Geometry: final body of the model. Coordinates: model frame, mm. Face numbers are marked on the shaded views. A direction names the side the tool comes from. Round coordinates to 2 decimals unless told otherwise and drop trailing zeros. Write each loop counter-clockwise with the first axis right and the second up, starting at its lowest first coordinate (ties: lowest second). Pieces come first, ordered by that corner, then holes. Notation, with made-up numbers: M 51.25,-16 L 84.25,-16 A30 ccw 84.25,21 Z; hole C -40,55.25 d9. An arc over 180 degrees is marked long. Answer as CSV lines item,"result". Start each with the question number.
Q1. Section query D-D on z = 10. Output: boundary loops of the cut face in (x, y).
Q2. Reachability of the marked faces 4 and 5 from +Z, -Z, +X, -X, +Y, -Y: full face, straight path, thin tool, end or side. Return the list, or none.
Q3. Section query B-B on z = 32.5. Output: boundary loops of the cut face in (x, y), and give its area (3 significant figures).
Q4. Section query C-C on x = 27. Output: boundary loops of the cut face in (y, z) (3 decimals).
Q5. Section query A-A on y = 12.7. Output: boundary loops of the cut face in (x, z) (3 decimals).
Q6. Mould query, pull axis Y, two halves, no side actions, for the marked faces 1, 2 and 3. Classes: pulls with the +Y half, pulls with the -Y half, needs draft (parallel to the pull), parting line crosses it, or undercut.
Q7. Ray query, probe 1 along Z at (x, y) = (20, 9) (3 decimals); probe 2 along Y at (x, z) = (30.48, 38.25); probe 3 along X at (y, z) = (12, 40). Return the intervals inside material, ascending.
Q8. First-contact query: pin 1 (6 mm diameter, centred on y = 22.5, z = 5, fed in from +X). Flat tip, straight axial feed; report the tip coordinate or a pass-through.
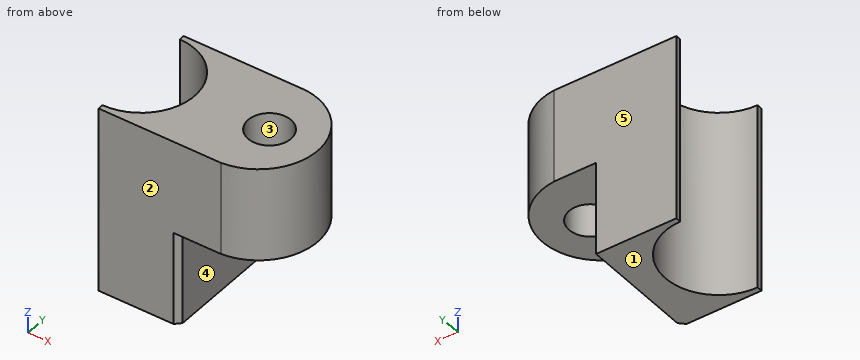
```python
from build123d import *

# Parameters (mm, degrees)
BOSS_EXTRUDE1_DEPTH          = 44.45
CUT_EXTRUDE1_DEPTH           = 22.225
F_3_8_0_375_DIAMETER_HOLE1_D = 10.16
CHAMFER1_SIZE                = 1.27


with BuildPart() as part:
    # Sketch1 → Boss-Extrude1 (new body)
    with BuildSketch(Plane.XY):
        with BuildLine():
            Line((0, -1.27), (29.046742048, -1.27))
            ThreePointArc((29.046742048, -1.27), (41.91, 12.7), (29.046742048, 26.67))
            Line((29.046742048, 26.67), (0, 26.67))
            Line((0, 26.67), (0, 25.4))
            ThreePointArc((0, 25.4), (12.7, 12.7), (0, 0))
            Line((0, 0), (0, -1.27))
        make_face()
    extrude(amount=BOSS_EXTRUDE1_DEPTH)

    # Sketch2 → Cut-Extrude1 (cut)
    with BuildSketch(Plane(origin=(0, 0, 0), x_dir=(-1, 0, 0), z_dir=(0, 0, -1))):
        with BuildLine():
            Line((-19.05, -1.27), (-19.05, 26.67))
            Line((-19.05, 26.67), (-29.046742048, 26.67))
            ThreePointArc((-29.046742048, 26.67), (-41.91, 12.7), (-29.046742048, -1.27))
            Line((-29.046742048, -1.27), (-19.05, -1.27))
        make_face()
    extrude(amount=-CUT_EXTRUDE1_DEPTH, mode=Mode.SUBTRACT)

    # 3/8 (0.375) Diameter Hole1 (through all)
    with Locations(Plane.XY.offset(44.45)):
        with Locations((30.48, 12.7)):
            Hole(F_3_8_0_375_DIAMETER_HOLE1_D / 2)

    # Chamfer1
    chamfer1_edges = [part.edges().sort_by_distance(p)[0] for p in [
        (19.05, -1.27, 11.1125),
    ]]
    chamfer(chamfer1_edges, length=CHAMFER1_SIZE)


solid = part.part
```
Entries:
1,outline,"M 0,-1.27 L 17.78,-1.27 L 19.05,0 L 19.05,26.67 L 0,26.67 L 0,25.4 A12.7 cw 0,0 Z"
2,face 4,"-Z, +X, +Y, -Y"
2,face 5,"+Z, -Z, +X, -X, +Y"
3,outline,"M 0,-1.27 L 29.05,-1.27 A14.02 ccw 29.05,26.67 L 0,26.67 L 0,25.4 A12.7 cw 0,0 Z; hole C 30.48,12.7 d10.16"
3,area,"753 mm^2"
4,outline,"M -1.27,22.225 L 8.999,22.225 L 8.999,44.45 L -1.27,44.45 Z; M 16.401,22.225 L 26.67,22.225 L 26.67,44.45 L 16.401,44.45 Z"
5,outline,"M 12.7,0 L 19.05,0 L 19.05,22.225 L 25.4,22.225 L 25.4,44.45 L 12.7,44.45 Z; M 35.56,22.225 L 41.91,22.225 L 41.91,44.45 L 35.56,44.45 Z"
6,face 1,"needs draft"
6,face 2,"pulls with the -Y half"
6,face 3,"undercut"
7,probe 1,"z = 22.225 to 44.45"
7,probe 2,"y = -1.08 to 7.62, 17.78 to 26.48"
7,probe 3,"x = 12.68 to 25.45, 35.51 to 41.89"
8,pin 1,"stops at x = 19.05"
